Part model, mm, in its own coordinate system. Round coordinates to 2 decimals unless told otherwise and drop trailing zeros. Loops run counter-clockwise (first coordinate to the right, second up) from the corner with the lowest first, then second, coordinate; pieces in that order, holes last. Notation, with made-up numbers: M -14.5,84 L 37.5,84 A34 cw 37.5,120 Z; hole C 24,15.5 d6. An arc over 180 degrees is marked long. Write each question's results on one line, items separated by ' | '.
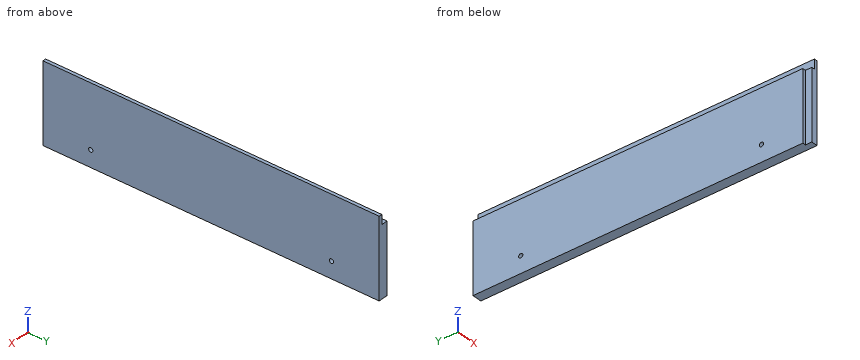
from build123d import *

# Parameters (mm, degrees)
SKETCH032_W             = 634
SKETCH032_H             = 150
PAD012_DEPTH            = 18
SKETCH033_W             = 634
SKETCH033_H             = 18
POCKET020_DEPTH         = 12
SKETCH034_W             = 12
SKETCH034_H             = 150
POCKET021_DEPTH         = 6
SKETCH040_R             = 4
POCKET024_DEPTH         = 18
BODY011_ROLL_ANGLE      = -90
BODY011_PLACEMENT_ANGLE = 90


with BuildPart() as part:
    # Sketch032 → Pad012 (new body)
    with BuildSketch(Plane.XY):
        with Locations((0, 75)):
            Rectangle(SKETCH032_W, SKETCH032_H)
    extrude(amount=PAD012_DEPTH)

    # Sketch033 (on Face6 of Pad012) → Pocket020 (cut)
    with BuildSketch(Plane.XY.offset(18)):
        with Locations((0, 9)):
            Rectangle(SKETCH033_W, SKETCH033_H)
    extrude(amount=-POCKET020_DEPTH, mode=Mode.SUBTRACT)

    # Sketch034 (on Face5 of Pocket020) → Pocket021 (cut)
    with BuildSketch(Plane.XY.offset(18)):
        with Locations((-311, 75)):
            Rectangle(SKETCH034_W, SKETCH034_H)
    extrude(amount=-POCKET021_DEPTH, mode=Mode.SUBTRACT)

    # Sketch040 (on Face2 of Pocket021) → Pocket024 (cut)
    with BuildSketch(Plane(origin=(0, 0, 0), x_dir=(1, 0, 0), z_dir=(0, 0, -1))):
        with Locations((-227, -118.5)):
            Circle(SKETCH040_R)
    pocket024 = extrude(amount=-POCKET024_DEPTH, mode=Mode.SUBTRACT)

    # Mirrored009: Pocket024 across Sketch040 V_Axis
    add(pocket024.mirror(Plane(origin=(0, 0, 0), x_dir=(0, 0, -1), z_dir=(1, 0, 0))), mode=Mode.SUBTRACT)


with BuildPart() as part_1:
    # Body011 roll: moved
    add(part.part.rotate(Axis((0, 0, 0), (1, 0, 0)), BODY011_ROLL_ANGLE))


with BuildPart() as part_2:
    # Body011 placement: moved
    add(part_1.part.moved(Location((263, 323, 150))).rotate(Axis((263, 323, 150), (0, 0, 1)), BODY011_PLACEMENT_ANGLE))


solid = part_2.part
Item 1: Band-saw the part on B-B on x = 253.75. Give the cut face in (y, z).
Filled sheet:
outline: M 6,0 L 640,0 L 640,132 L 6,132 Z; hole C 96,31.5 d8; hole C 550,31.5 d8
Item 2: Band-saw the part on A-A on y = 510.5. Give the cut face in (x, z), and give its area (3 significant figures).
Filled sheet:
outline: M 245,0 L 263,0 L 263,150 L 257,150 L 257,132 L 245,132 Z | area: 2,480 mm^2
Item 3: Drop flat-ended pins along their axis: P1, Ø3, axis at x = 249, z = 83.5, coming from the -Y side; P2, Ø4, axis at x = 253, y = 545, coming from the +Z side; P3, Ø9, axis at y = 185.5, z = 142, coming from the -X side; P4, Ø7, axis at y = 550, z = 31.5, coming from the -X side. Give the stop position or say it passes through.
Filled sheet:
P1: y = 18 | P2: z = 132 | P3: x = 257 | P4: through
Item 4: Wall check: L1, parallel to Z at x = 255.5, y = 96; L2, parallel to Z at x = 254, y = 54; L3, parallel to Y at x = 248.25, z = 93. Give the ranges that are in metal, low to high.
Filled sheet:
L1: 0 to 27.5, 35.5 to 132 | L2: 0 to 132 | L3: 18 to 640
